Source: three-view drawing plus pictorial views. Frame: mm from the lowest corner of the part. A direction names the side the tool comes from. Give positions to 0.01 mm unless a question says otherwise; leave off trailing zeros. Loops run counter-clockwise (first coordinate to the right, second up) from the corner with the lowest first, then second, coordinate; pieces in that order, holes last. Notation, with made-up numbers: M 30.5,-12 L 64.5,-12 A16 ccw 64.5,4 Z; hole C 1.5,-34 d8. An arc over 180 degrees is marked long. One line per item, written item: value. Start each with the question number.
(1) Section B-B on y = 43. Output: boundary loops of the cut face in (x, z).
(2) Pin query (flat end, axial travel): P1, Ø12, axis at x = 13.5, z = 42, coming from the +Y side; P2, Ø1.8, axis at x = 7.5, y = 5, coming from the +Z side; P3, Ø2, axis at x = 19.5, z = 22, coming from the -Y side; P4, Ø3.5, axis at x = 20, y = 81, coming from the +Z side. Return the tip coordinate at first contact, or that it passes through.
(3) Ray query, line 1 along Y through (x, z) = (3.9, 4.5); line 2 along Y through (x, z) = (7.5, 1.95); line 3 along Y through (x, z) = (1.1, 51.5). Return the intervals inside material, ascending. Write a range as from..to.
(4) Section D-D on x = 28.5. Output: boundary loops of the cut face in (y, z).
(5) Access query for the marked faces 5, 6 and 7. Directions: +Z, -Z, +X, -X, +Y, -Y. A direction counts if a zero-diameter tool reaches every point of the face in a straight line with its end or side. Return the directions, or none.
(6) Section A-A on x = 7.5. Output: boundary loops of the cut face in (y, z), plus the area to 3 significant figures.
(7) Pull-direction query (Y, two-part tool) for the marked faces 1, 2, 3 and 4; classes: released by +Y, released by -Y, zero draft, split by the parting line, or undercut.
(8) Section C-C on z = 45. Output: boundary loops of the cut face in (x, y), plus the area to 3 significant figures.
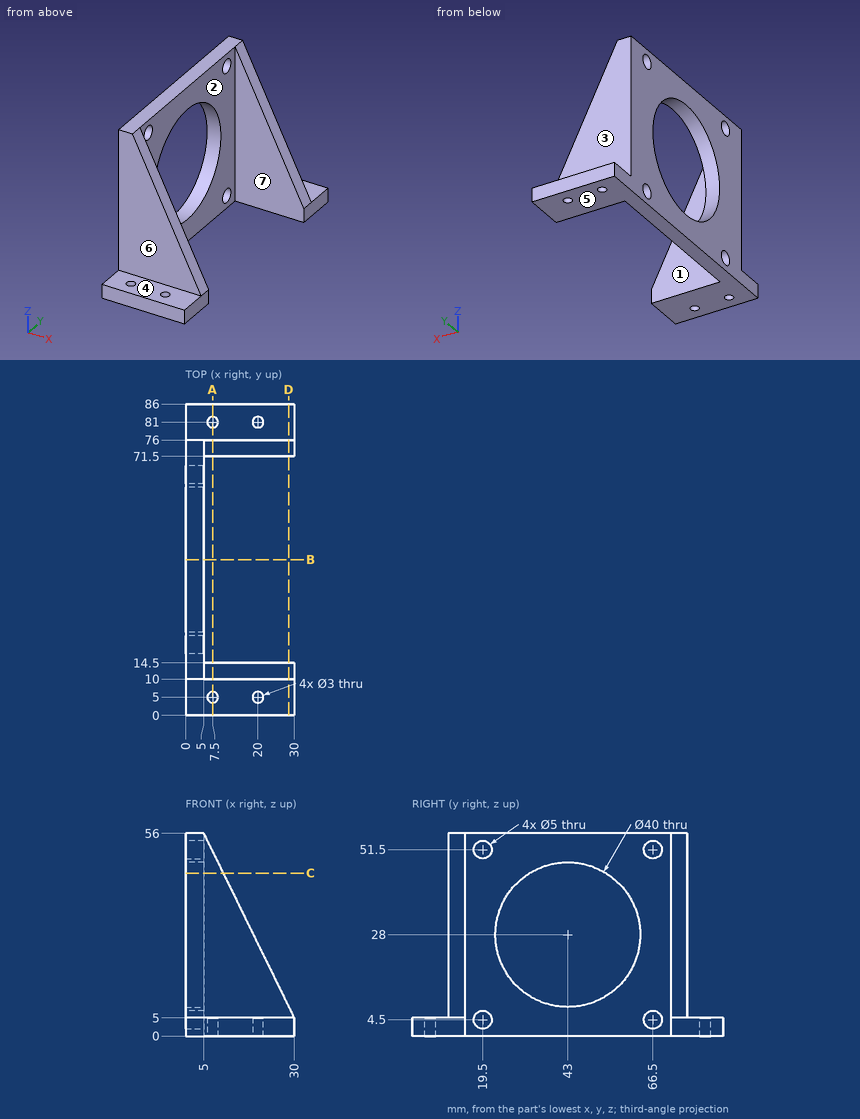
Output values:
1. outline: M 0,0 L 5,0 L 5,8 L 0,8 Z; M 0,48 L 5,48 L 5,56 L 0,56 Z
2. P1: stops at y = 76
2. P2: passes through
2. P3: stops at y = 10
2. P4: stops at z = 5
3. line 1: y = 0..17, 22..64, 69..86
3. line 2: y = 0..3.5, 6.5..14.5, 71.5..79.5, 82.5..86
3. line 3: y = 10..17, 22..64, 69..76
4. outline: M 0,0 L 14.5,0 L 14.5,8.06 L 10,8.06 L 10,5 L 0,5 Z; M 71.5,0 L 86,0 L 86,5 L 76,5 L 76,8.06 L 71.5,8.06 Z
5. face 5: -Z, +X, -X, +Y, -Y
5. face 6: +Z, +X, -X, -Y
5. face 7: +Z, -Z, +X
6. outline: M 0,0 L 3.5,0 L 3.5,5 L 0,5 Z; M 6.5,0 L 14.5,0 L 14.5,50.9 L 10,50.9 L 10,5 L 6.5,5 Z; M 71.5,0 L 79.5,0 L 79.5,5 L 76,5 L 76,50.9 L 71.5,50.9 Z; M 82.5,0 L 86,0 L 86,5 L 82.5,5 Z
6. area: 528 mm²
7. face 1: undercut
7. face 2: undercut
7. face 3: released by +Y
7. face 4: zero draft
8. outline: M 0,10 L 10.39,10 L 10.39,14.5 L 5,14.5 L 5,32.46 L 0,32.46 Z; M 0,53.54 L 5,53.54 L 5,71.5 L 10.39,71.5 L 10.39,76 L 0,76 Z
8. area: 273 mm²
